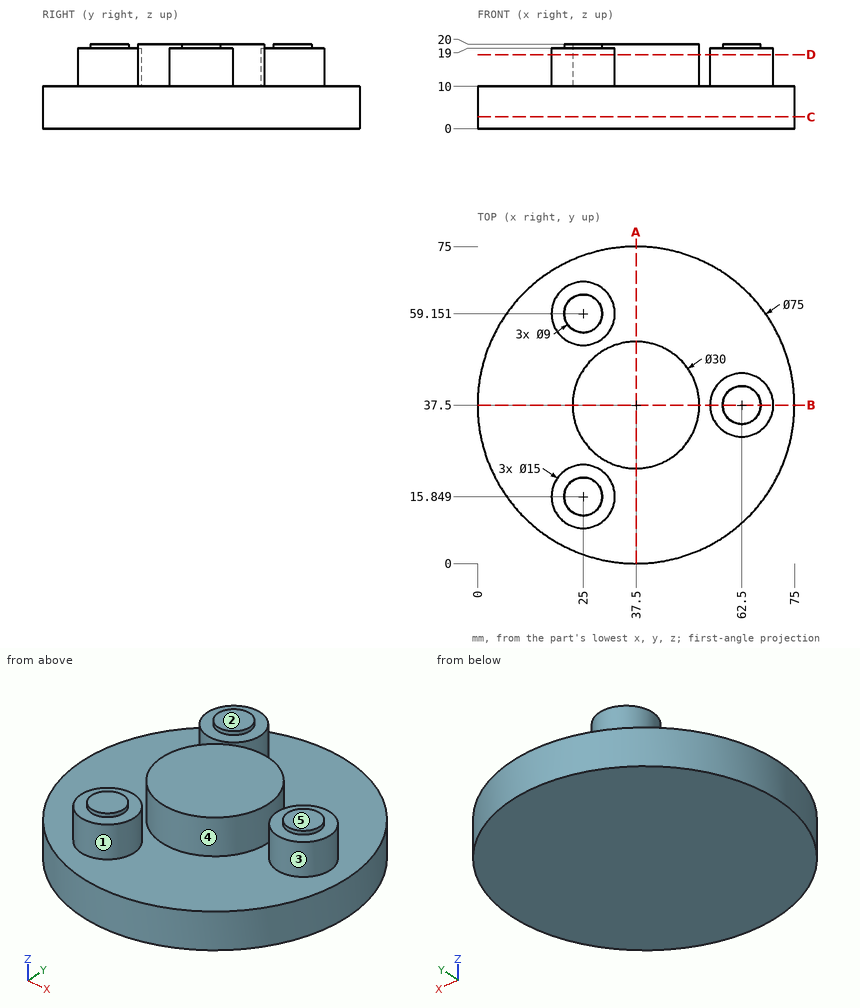
For this review, use the dimensioned drawing (mm, ordinates from the lowest corner) and the shaded views. A direction names the side the tool comes from. Round coordinates to 2 decimals unless told otherwise and drop trailing zeros. Order: outer loops, then holes, each group sorted by start corner. A loop starts at its lowest first (then second) coordinate and runs counter-clockwise, first axis right, second up. Notation, with made-up numbers: M -20,82.25 L 7,82.25 A13 ccw 7,98.25 Z; hole C 48.25,-39 d11. An arc over 180 degrees is marked long. Use a Markdown table: item, result. Add a question column.
Item 1: Add section A-A, the plane x = 37.5. Give the boundary of the cut face in (y, z).
Item 2: Tool access review of the marked faces 4 and 5: name each direction out of +Z, -Z, +X, -X, +Y, -Y from which nothing blocks a thin tool from reaching the whole face with its end or side.
Item 3: Add section D-D, the plane z = 17.5. Give the boundary of the cut face in (x, y), then the cut area to 3 significant figures.
Item 4: Insertion check: pin 1 (10 mm diameter, centred on x = 59.5, y = 21.5, fed in from -Z); pin 2 (10 mm diameter, centred on x = 64.5, z = 5.5, fed in from -Y); pin 3 (12 mm diameter, centred on x = 49, z = 7, fed in from -Y) (1 decimal); pin 4 (10 mm diameter, centred on x = 47.5, z = 6.5, fed in from +Y) (1 decimal). Each pin has a flat end and moves straight along its axis. Give the tip position at first contact, or say it passes through.
Item 5: Mouldability with a two-part tool opening along Y and no side actions: class the marked faces 1, 2 and 3 as released by +Y, released by -Y, zero draft, split by the parting line, or undercut.
Item 6: Add section C-C, the plane z = 2.75. Give the boundary of the cut face in (x, y).
Item 7: Add section B-B, the plane y = 37.5. Give the boundary of the cut face in (x, z), then the cut area to 3 significant figures.
Item 8: To check wall thickness, follow line 1 along Y through (x, z) = (27, 14); line 2 along Y through (x, z) = (30, 13.5); line 3 along Y through (x, z) = (37, 6.75). State the ranges of each line that lie inside material, in increasing order.
Geometry results:
| question | item | result |
|---|---|---|
| 1 | outline | M 0,0 L 75,0 L 75,10 L 52.5,10 L 52.5,20 L 22.5,20 L 22.5,10 L 0,10 Z |
| 2 | face 4 | +Z |
| 2 | face 5 | +Z, +X, -X, +Y, -Y |
| 3 | outline | C 25,15.85 d15; C 25,59.15 d15; C 37.5,37.5 d30; C 62.5,37.5 d15 |
| 3 | area | 1,240 mm² |
| 4 | pin 1 | stops at z = 0 |
| 4 | pin 2 | stops at y = 7.13 |
| 4 | pin 3 | stops at y = 0.4 |
| 4 | pin 4 | stops at y = 74.7 |
| 5 | face 1 | undercut |
| 5 | face 2 | zero draft |
| 5 | face 3 | split by the parting line |
| 6 | outline | C 37.5,37.5 d75 |
| 7 | outline | M 0,0 L 75,0 L 75,10 L 70,10 L 70,19 L 67,19 L 67,20 L 58,20 L 58,19 L 55,19 L 55,10 L 52.5,10 L 52.5,20 L 22.5,20 L 22.5,10 L 0,10 Z |
| 7 | area | 1,190 mm² |
| 8 | line 1 | y = 8.62 to 23.08, 26.79 to 48.21, 51.92 to 66.38 |
| 8 | line 2 | y = 10.26 to 21.44, 24.51 to 50.49, 53.56 to 64.74 |
| 8 | line 3 | y = 0 to 75 |
